Build history of the part. All positions in model axes, mm. A direction names the side the tool comes from. Coordinates: 2 decimals unless noted, no trailing zeros. Write each loop counter-clockwise with the first axis right and the second up, starting at its lowest first coordinate (ties: lowest second). Pieces come first, ordered by that corner, then holes. Notation, with made-up numbers: (10, 13.25) -> (58, 13.25) arc R15 ccw to (58, 30.25) -> close; hole circle Ø5 at (24, -7). An arc over 180 degrees is marked (long way). Write each question's results on one line, items separated by ' | '. Start each with the question number.
Q1. Tool access for faces 5 (the face through (13.53, -13.51, -16.48)), 6 (the face through (14.25, 0, -16)), 7 (the face through (0, -14.25, -16)), 8 (the face through (1.107, -8.428, 25.044)), 9 (the face through (-4, 2, 25.5)): list every direction of +Z, -Z, +X, -X, +Y, -Y with a clear straight run to the whole face (end or side of a thin tool).
Q2. Drill centre lines: line 1 (Y direction, x = 0, z = 22.75); line 2 (Y direction, x = 11.5, z = 19.4); line 3 (Y direction, x = 0, z = -31.9). Where is each one in solid material? Low to high.
Q3. Drop flat-ended pins along their axis: pin 1 Ø2 at (x, y) = (0, 5) entering from +Z; pin 2 Ø2.5 at (x, y) = (-2, -2) entering from -Z; pin 3 Ø8 at (x, z) = (-1, -9) entering from +Y. Give the stop position or say it passes through.
Q4. Saw through at B-B on z = -19.5. Give the cut face in (x, y).
Q5. Saw through at C-C on y = 7.5. Give the cut face in (x, z).
Q6. Saw through at D-D on z = 4. Give the cut face in (x, y).
Q7. Two-plate mould, pull along X, no slides. Class faces 1 (the face through (-6.25, 0.05, 23.39)), 2 (the face through (0.12, -4.82, 20.88)), 3 (the face through (0, 15, 11)), 4 (the face through (-10.316, -7.91, 23.586)): released by +X, released by -X, zero draft, split by the parting line, or undercut.
Q8. Saw through at A-A on z = 19.5. Give the cut face in (x, y), and give its area (3 significant figures).
from build123d import *

# Parameters (mm, degrees)
SKETCH1_W           = 30
SKETCH1_H           = 30
BOSS_EXTRUDE1_DEPTH = 22.6
SKETCH3_W           = 28.5
SKETCH3_H           = 28.5
BOSS_EXTRUDE2_DEPTH = 32.5
SKETCH4_R           = 13
BOSS_EXTRUDE3_DEPTH = 2
SKETCH5_R           = 8.5
BOSS_EXTRUDE4_DEPTH = 0.9
SKETCH6_R           = 3
SKETCH6_R_2         = 1.25
CUT_EXTRUDE1_DEPTH  = 4
SKETCH10_R          = 1.25
CUT_EXTRUDE2_DEPTH  = 5
SKETCH12_R          = 3
CUT_EXTRUDE3_DEPTH  = 1
SKETCH13_R          = 29.849433241
SKETCH13_R_2        = 19.849433241
CUT_EXTRUDE4_DEPTH  = 22.6
SKETCH14_R          = 22.5
SKETCH14_R_2        = 19.121323176
CUT_EXTRUDE5_DEPTH  = 32.5
SKETCH15_R          = 4.5
CUT_EXTRUDE6_DEPTH  = 1
BOSS_EXTRUDE5_START = -1
SKETCH16_W          = 12
SKETCH16_H          = 0.75
BOSS_EXTRUDE5_DEPTH = 3


# Read off the part's stored shape, not the designer's step: M3x0.5 Tapped Hole1, M3x0.5 Tapped Hole2
with BuildPart() as part:
    # Sketch1 → Boss-Extrude1 (new body)
    with BuildSketch(Plane.XY):
        Rectangle(SKETCH1_W, SKETCH1_H)
    extrude(amount=BOSS_EXTRUDE1_DEPTH)

    # Sketch3 → Boss-Extrude2 (add)
    with BuildSketch(Plane(origin=(0, 0, 0), x_dir=(-1, 0, 0), z_dir=(0, 0, -1))):
        Rectangle(SKETCH3_W, SKETCH3_H)
    extrude(amount=BOSS_EXTRUDE2_DEPTH)

    # Sketch4 → Boss-Extrude3 (add)
    with BuildSketch(Plane.XY.offset(22.6)):
        Circle(SKETCH4_R)
    extrude(amount=BOSS_EXTRUDE3_DEPTH)

    # Sketch5 → Boss-Extrude4 (add)
    with BuildSketch(Plane.XY.offset(24.6)):
        with Locations(Location((0, 0, 0), (0, 0, 180))):
            Circle(SKETCH5_R)
    extrude(amount=BOSS_EXTRUDE4_DEPTH)

    # Sketch6 → Cut-Extrude1 (cut)
    with BuildSketch(Plane.XY.offset(25.5)):
        Circle(SKETCH6_R)
        with Locations((0, 5)):
            Circle(SKETCH6_R_2)
        with Locations((5, 0)):
            Circle(SKETCH6_R_2)
        with Locations((0, -5)):
            Circle(SKETCH6_R_2)
        with Locations((-5, 0)):
            Circle(SKETCH6_R_2)
    extrude(amount=-CUT_EXTRUDE1_DEPTH, mode=Mode.SUBTRACT)

    # M3x0.5 Tapped Hole1 outline → M3x0.5 Tapped Hole1 (revolve, cut)
    with BuildSketch(Plane(origin=(-5, 0, 0), x_dir=(1, 0, 0), z_dir=(0, -1, 0))):
        Polygon((1.25, 25.5), (1.25, 25.225), (1.525, 25.5), align=None)
    revolve(axis=Axis((-5, 0, 0), (0, 0, 1)), mode=Mode.SUBTRACT)

    # M3x0.5 Tapped Hole1 2 outline → M3x0.5 Tapped Hole1 2 (revolve, cut)
    with BuildSketch(Plane.XZ.offset(5)):
        Polygon((1.25, 25.5), (1.25, 25.225), (1.525, 25.5), align=None)
        Polygon((0, 20.748924226), (1.25, 21.5), (0, 21.5), align=None)
    revolve(axis=Axis((0, -5, 0), (0, 0, 1)), mode=Mode.SUBTRACT)

    # M3x0.5 Tapped Hole1 3 outline → M3x0.5 Tapped Hole1 3 (revolve, cut)
    with BuildSketch(Plane(origin=(5, 0, 0), x_dir=(1, 0, 0), z_dir=(0, -1, 0))):
        Polygon((1.25, 25.5), (1.25, 25.225), (1.525, 25.5), align=None)
        Polygon((0, 20.748924226), (1.25, 21.5), (0, 21.5), align=None)
    revolve(axis=Axis((5, 0, 0), (0, 0, 1)), mode=Mode.SUBTRACT)

    # M3x0.5 Tapped Hole1 4 outline → M3x0.5 Tapped Hole1 4 (revolve, cut)
    with BuildSketch(Plane.XZ.offset(-5)):
        Polygon((1.25, 25.5), (1.25, 25.225), (1.525, 25.5), align=None)
        Polygon((0, 20.748924226), (1.25, 21.5), (0, 21.5), align=None)
    revolve(axis=Axis((0, 5, 0), (0, 0, 1)), mode=Mode.SUBTRACT)

    # Sketch10 → Cut-Extrude2 (cut)
    with BuildSketch(Plane.XY.offset(22.6)):
        with Locations((-11.5, -11.5)):
            Circle(SKETCH10_R)
        with Locations((-11.5, 11.5)):
            Circle(SKETCH10_R)
        with Locations((11.5, 11.5)):
            Circle(SKETCH10_R)
        with Locations((11.5, -11.5)):
            Circle(SKETCH10_R)
    extrude(amount=-CUT_EXTRUDE2_DEPTH, mode=Mode.SUBTRACT)

    # M3x0.5 Tapped Hole2 outline → M3x0.5 Tapped Hole2 (revolve, cut)
    with BuildSketch(Plane(origin=(-11.5, -11.5, 0), x_dir=(1, 0, 0), z_dir=(0, -1, 0))):
        Polygon((1.25, 22.6), (1.25, 22.325), (1.525, 22.6), align=None)
    revolve(axis=Axis((-11.5, -11.5, 0), (0, 0, 1)), mode=Mode.SUBTRACT)

    # M3x0.5 Tapped Hole2 2 outline → M3x0.5 Tapped Hole2 2 (revolve, cut)
    with BuildSketch(Plane(origin=(11.5, -11.5, 0), x_dir=(1, 0, 0), z_dir=(0, -1, 0))):
        Polygon((1.25, 22.6), (1.25, 22.325), (1.525, 22.6), align=None)
        Polygon((0, 16.848924226), (1.25, 17.6), (0, 17.6), align=None)
    revolve(axis=Axis((11.5, -11.5, 0), (0, 0, 1)), mode=Mode.SUBTRACT)

    # M3x0.5 Tapped Hole2 3 outline → M3x0.5 Tapped Hole2 3 (revolve, cut)
    with BuildSketch(Plane(origin=(11.5, 11.5, 0), x_dir=(1, 0, 0), z_dir=(0, -1, 0))):
        Polygon((1.25, 22.6), (1.25, 22.325), (1.525, 22.6), align=None)
        Polygon((0, 16.848924226), (1.25, 17.6), (0, 17.6), align=None)
    revolve(axis=Axis((11.5, 11.5, 0), (0, 0, 1)), mode=Mode.SUBTRACT)

    # M3x0.5 Tapped Hole2 4 outline → M3x0.5 Tapped Hole2 4 (revolve, cut)
    with BuildSketch(Plane(origin=(-11.5, 11.5, 0), x_dir=(1, 0, 0), z_dir=(0, -1, 0))):
        Polygon((1.25, 22.6), (1.25, 22.325), (1.525, 22.6), align=None)
        Polygon((0, 16.848924226), (1.25, 17.6), (0, 17.6), align=None)
    revolve(axis=Axis((-11.5, 11.5, 0), (0, 0, 1)), mode=Mode.SUBTRACT)

    # Sketch12 → Cut-Extrude3 (cut)
    with BuildSketch(Plane.XZ.offset(15)):
        with Locations(Location((0, 4, 0), (0, 0, 270))):
            Circle(SKETCH12_R)
    extrude(amount=-CUT_EXTRUDE3_DEPTH, mode=Mode.SUBTRACT)

    # Sketch13 → Cut-Extrude4 (cut)
    with BuildSketch(Plane.XY.offset(22.6)):
        Circle(SKETCH13_R)
        Circle(SKETCH13_R_2, mode=Mode.SUBTRACT)
    extrude(amount=-CUT_EXTRUDE4_DEPTH, mode=Mode.SUBTRACT)

    # Sketch14 → Cut-Extrude5 (cut)
    with BuildSketch(Plane(origin=(0, 0, -32.5), x_dir=(-1, 0, 0), z_dir=(0, 0, -1))):
        Circle(SKETCH14_R)
        Circle(SKETCH14_R_2, mode=Mode.SUBTRACT)
    extrude(amount=-CUT_EXTRUDE5_DEPTH, mode=Mode.SUBTRACT)

    # Sketch15 → Cut-Extrude6 (cut)
    with BuildSketch(Plane(origin=(0, 0, -32.5), x_dir=(-1, 0, 0), z_dir=(0, 0, -1))):
        Circle(SKETCH15_R)
    extrude(amount=-CUT_EXTRUDE6_DEPTH, mode=Mode.SUBTRACT)

    # Sketch16 → Boss-Extrude5 (add)
    with BuildSketch(Plane(origin=(0, 0, -32.5), x_dir=(-1, 0, 0), z_dir=(0, 0, -1)).offset(BOSS_EXTRUDE5_START)):
        with Locations((0, 14.625)):
            Rectangle(SKETCH16_W, SKETCH16_H)
    extrude(amount=-BOSS_EXTRUDE5_DEPTH)


solid = part.part
Returned:
1) face 5: -Z, +X, -Y | face 6: -Z, +X, +Y, -Y | face 7: -Z, +X, -X, -Y | face 8: +Z | face 9: +Z, +X, -X, +Y, -Y
2) line 1: y = -13 to -6.25, -3.75 to -3, 3 to 3.75, 6.25 to 13 | line 2: y = -15 to -12.75, -10.25 to 10.25, 12.75 to 15 | line 3: y = -14.25 to -4.5, 4.5 to 14.25
3) pin 1: stops at z = 21.35 | pin 2: stops at z = -31.5 | pin 3: stops at y = 14.25
4) outline: (-14.25, -12.75) arc R19.12 ccw to (-12.75, -14.25) -> (12.75, -14.25) arc R19.12 ccw to (14.25, -12.75) -> (14.25, 12.75) arc R19.12 ccw to (12.75, 14.25) -> (-12.75, 14.25) arc R19.12 ccw to (-14.25, 12.75) -> close
5) outline: (-15, 0) -> (-14.25, 0) -> (-14.25, -32.5) -> (14.25, -32.5) -> (14.25, 0) -> (15, 0) -> (15, 22.6) -> (10.62, 22.6) -> (10.62, 24.6) -> (4, 24.6) -> (4, 25.5) -> (-4, 25.5) -> (-4, 24.6) -> (-10.62, 24.6) -> (-10.62, 22.6) -> (-15, 22.6) -> close
6) outline: (-15, -13) arc R19.85 ccw to (-13, -15) -> (-3, -15) -> (-3, -14) -> (3, -14) -> (3, -15) -> (13, -15) arc R19.85 ccw to (15, -13) -> (15, 13) arc R19.85 ccw to (13, 15) -> (-13, 15) arc R19.85 ccw to (-15, 13) -> close
7) face 1: undercut | face 2: undercut | face 3: zero draft | face 4: split by the parting line
8) outline: (-15, -13) arc R19.85 ccw to (-13, -15) -> (13, -15) arc R19.85 ccw to (15, -13) -> (15, 13) arc R19.85 ccw to (13, 15) -> (-13, 15) arc R19.85 ccw to (-15, 13) -> close; hole circle Ø2.5 at (-11.5, -11.5); hole circle Ø2.5 at (-11.5, 11.5); hole circle Ø2.5 at (11.5, -11.5); hole circle Ø2.5 at (11.5, 11.5) | area: 873 mm2
